Here's how the part is built. I have some questions about the finished solid (model axes, mm). A direction names the side the tool comes from. Give positions to 0.01 mm unless a question says otherwise; leave off trailing zeros. Write each loop counter-clockwise with the first axis right and the second up, starting at its lowest first coordinate (ties: lowest second). Pieces come first, ordered by that corner, then holes. Notation, with made-up numbers: (70.5, -16.5) -> (77.5, -16.5) arc R23 cw to (77.5, 4.5) -> close; hole circle Ø6 at (7.5, 62). An arc over 180 degrees is marked (long way). Use one line per item in the form item = value.
```python
from build123d import *
from build123d.topology import SkipClean

# Parameters (mm, degrees)
EXTRUDE_1_DEPTH     = 0.8
SKETCH_2_R          = 6.4
EXTRUDE_2_DEPTH     = 4
EXTRUDE_3_DEPTH     = 8
CUT_EXTRUDE_1_REACH = 22.508
SKETCH_4_R          = 6.4
SKETCH_5_R          = 0.85
CUT_EXTRUDE_2_DEPTH = 21.508362032


# Read off the part's stored shape, not the designer's step: 填料-伸長3
with BuildPart() as part:
    # 草圖1 → 填料-伸長1 (new body)
    with BuildSketch(Plane(origin=(0, 0, 0), x_dir=(1, 0, 0), z_dir=(0, 1, 0))):
        with BuildLine():
            Line((7, 6.586363636), (7, -7.413636364))
            ThreePointArc((7, -7.413636364), (0, -14.413636364), (-7, -7.413636364))
            Line((-7, -7.413636364), (-7, 6.586363636))
            ThreePointArc((-7, 6.586363636), (0, 13.586363636), (7, 6.586363636))
        make_face()
    extrude(amount=EXTRUDE_1_DEPTH)

    # 草圖2 → 填料-伸長2 (add)
    with SkipClean():  # the faces are left unmerged after this step: merging them gives an invalid solid
        with BuildSketch(Plane(origin=(0, 0.8, 0), x_dir=(1, 0, 0), z_dir=(0, 1, 0))):
            with BuildLine():
                Line((5, -2.514656878), (5, 1.687384151))
                ThreePointArc((5, 1.687384151), (0, 13.586363636), (-5, 1.687384151))
                Line((-5, 1.687384151), (-5, -2.514656878))
                ThreePointArc((-5, -2.514656878), (0, -14.413636364), (5, -2.514656878))
            make_face()
            with Locations(Location((0, 6.586363636, 0), (0, 0, 270))):
                Circle(SKETCH_2_R, mode=Mode.SUBTRACT)
            with Locations(Location((0, -7.413636364, 0), (0, 0, 270))):
                Circle(SKETCH_2_R, mode=Mode.SUBTRACT)
        extrude(amount=EXTRUDE_2_DEPTH)

    # 填料-伸長3 outline → 填料-伸長3 (add)
    with SkipClean():  # the faces are left unmerged after this step: merging them gives an invalid solid
        with BuildSketch(Plane(origin=(0, 4.8, 0), x_dir=(1, 0, 0), z_dir=(0, 1, 0))):
            with BuildLine():
                ThreePointArc((5, 1.687384151), (0, 13.586363636), (-5, 1.687384151))
                Line((-5, 1.687384151), (-5, -2.514656878))
                ThreePointArc((-5, -2.514656878), (0, -14.413636364), (5, -2.514656878))
                Line((5, -2.514656878), (5, 1.687384151))
            make_face()
        extrude(amount=EXTRUDE_3_DEPTH)

    # 草圖4 → 除料-伸長1 (cut, up to next)
    with BuildSketch(Plane.XZ, mode=Mode.PRIVATE) as cut_extrude_1_sk1:
        with Locations(Location((0, 7.413636364, 0), (0, 0, 270))):
            Circle(SKETCH_4_R)
    cut_extrude_1_tool1 = extrude(cut_extrude_1_sk1.sketch, amount=-CUT_EXTRUDE_1_REACH, mode=Mode.PRIVATE) & part.part
    # 草圖4 → 除料-伸長1 (cut, up to next)
    with BuildSketch(Plane.XZ, mode=Mode.PRIVATE) as cut_extrude_1_sk2:
        with Locations(Location((0, -6.586363636, 0), (0, 0, 270))):
            Circle(SKETCH_4_R)
    cut_extrude_1_tool2 = extrude(cut_extrude_1_sk2.sketch, amount=-CUT_EXTRUDE_1_REACH, mode=Mode.PRIVATE) & part.part
    add(cut_extrude_1_tool1.solids().sort_by_distance((0, 0, 7.413636))[0], mode=Mode.SUBTRACT)
    add(cut_extrude_1_tool2.solids().sort_by_distance((0, 0, -6.586364))[0], mode=Mode.SUBTRACT)

    # 草圖5 → 除料-伸長2 (cut, through all)
    with SkipClean():  # the faces are left unmerged after this step: merging them gives an invalid solid
        with BuildSketch(Plane(origin=(0, 12.8, 0), x_dir=(1, 0, 0), z_dir=(0, 1, 0))):
            with Locations(Location((-1.5, 8.086363636, 0), (0, 0, 270))):
                Circle(SKETCH_5_R)
            with Locations(Location((1.5, 8.086363636, 0), (0, 0, 270))):
                Circle(SKETCH_5_R)
            with Locations(Location((1.5, 5.086363636, 0), (0, 0, 270))):
                Circle(SKETCH_5_R)
            with Locations(Location((-1.5, 5.086363636, 0), (0, 0, 270))):
                Circle(SKETCH_5_R)
            with Locations(Location((1.5, -5.913636364, 0), (0, 0, 270))):
                Circle(SKETCH_5_R)
            with Locations(Location((1.5, -8.913636364, 0), (0, 0, 270))):
                Circle(SKETCH_5_R)
            with Locations(Location((-1.5, -5.913636364, 0), (0, 0, 270))):
                Circle(SKETCH_5_R)
            with Locations(Location((-1.5, -8.913636364, 0), (0, 0, 270))):
                Circle(SKETCH_5_R)
        extrude(amount=-CUT_EXTRUDE_2_DEPTH, mode=Mode.SUBTRACT)


solid = part.part
```
Q1. If I drill on line 1 along Z through (x, y) = (0, 0.3); line 2 along Z through (x, y) = (2.25, 10.25); line 3 along Z through (x, y) = (3.25, 1.5), over which ranges is the centre line in solid material (lowest first)? Write a range as from..to.
Result set:
line_1 = -13.59..-12.99, -0.19..1.01, 13.81..14.41
line_2 = -13.21..-8.49, -7.69..-5.49, -4.69..5.51, 6.31..8.51, 9.31..14.04
line_3 = -12.79..-12.1, -1.07..1.9, 12.93..13.61
Q2. I want a section at B-B, the plane z = -5. Write out the boundary of the cut face in (x, y).
Result set:
outline = (-7, 0) -> (-6.2, 0) -> (-6.2, 4.8) -> (-2.35, 4.8) -> (-2.35, 12.8) -> (-6.82, 12.8) -> (-6.82, 0.8) -> (-7, 0.8) -> close; (-0.65, 4.8) -> (0.65, 4.8) -> (0.65, 12.8) -> (-0.65, 12.8) -> close; (2.35, 4.8) -> (6.2, 4.8) -> (6.2, 0) -> (7, 0) -> (7, 0.8) -> (6.82, 0.8) -> (6.82, 12.8) -> (2.35, 12.8) -> close
Q3. I want a section at A-A, the plane y = 7. Count the separate pieces of the cut face and the enclosed holes in it, and give its area (3 significant figures).
Result set:
separate_pieces = 1
enclosed_holes = 8
area = 303 mm2
Q4. If we mould it in two halves opening along X, with no side actions, what happens to faces 1 (the face through (1, 0, 0)), 2 (the face through (-1.826, 8.856, 9.699)), 3 (the face through (-1.245, 8.856, -4.276))? For each: +X half, -X half, draft (parallel to the pull), parting line (faces both ways), or undercut.
Result set:
face_1 = draft
face_2 = undercut
face_3 = undercut
Q5. I want a section at D-D, the plane x = 0. Write out the boundary of the cut face in (y, z), and give its area (3 significant figures).
Result set:
outline = (0, -13.59) -> (12.8, -13.59) -> (12.8, 14.41) -> (0, 14.41) -> (0, 13.81) -> (4.8, 13.81) -> (4.8, 1.01) -> (0, 1.01) -> (0, -0.19) -> (4.8, -0.19) -> (4.8, -12.99) -> (0, -12.99) -> close
area = 236 mm2
Q6. Which directions (+Z, -Z, +X, -X, +Y, -Y) give clear straight access to the entire face, cutting with the end or side of a thin tool? Please do faces 4 (the face through (0, 12.8, 0)), 5 (the face through (1.174, 8.856, 9.699)), 6 (the face through (-6, 0.8, 0)), 7 (the face through (0, 4.8, 7)), 8 (the face through (6, 0.8, 0)).
Result set:
face_4 = +Z, -Z, +X, -X, +Y
face_5 = +Y, -Y
face_6 = -X, +Y
face_7 = -Y
face_8 = +X, +Y
Q7. Will these pins go through, and if not, where does the flat tip stop? pin 1 Ø2.5 at (x, z) = (-1.5, -5.09) entering from -Y; pin 2 Ø3 at (y, z) = (3.5, 0) entering from +X; pin 3 Ø3 at (x, y) = (3.5, 3) entering from +Z; pin 4 Ø1 at (x, z) = (-1.5, 5.91) entering from -Y.
Result set:
pin_1 = 4.8
pin_2 = 5
pin_3 = 14.12
pin_4 = through
Q8. I want a section at C-C, the plane x = 1.5. Write out the boundary of the cut face in (y, z).
Result set:
outline = (0, -13.42) -> (12.8, -13.42) -> (12.8, -8.94) -> (4.8, -8.94) -> (4.8, -12.81) -> (0, -12.81) -> close; (0, -0.36) -> (4.8, -0.36) -> (4.8, -4.24) -> (12.8, -4.24) -> (12.8, 5.06) -> (4.8, 5.06) -> (4.8, 1.19) -> (0, 1.19) -> close; (0, 13.64) -> (4.8, 13.64) -> (4.8, 9.76) -> (12.8, 9.76) -> (12.8, 14.25) -> (0, 14.25) -> close; (4.8, -7.24) -> (12.8, -7.24) -> (12.8, -5.94) -> (4.8, -5.94) -> close; (4.8, 6.76) -> (12.8, 6.76) -> (12.8, 8.06) -> (4.8, 8.06) -> close
